Source: CAD feature listing. Evaluate the final solid. Frame: model axes, mm. Face numbers are marked on the shaded views. Round coordinates to 2 decimals unless told otherwise and drop trailing zeros. Write each loop counter-clockwise with the first axis right and the second up, starting at its lowest first coordinate (ties: lowest second). Pieces come first, ordered by that corner, then holes. Notation, with made-up numbers: M 78.5,67.25 L 91.5,67.25 A12 cw 91.5,75.25 Z; hole C 49.25,20.5 d3. An arc over 180 degrees is marked long. Answer in a Markdown table with one row per item. Add a question column.
Item 1: Cut plane B-B on y = 7.5. Return loops of the section in (x, z), and give its area (3 significant figures).
Item 2: Cut plane A-A on x = 29. Return loops of the section in (y, z).
Item 3: Mould query, pull axis Y, two halves, no side actions, for the marked faces 1, 2 and 3. Classes: released by +Y, released by -Y, zero draft, split by the parting line, or undercut.
Item 4: Material intervals for probe 1 along X at (y, z) = (-14, 21.25); probe 2 along Z at (x, y) = (-7, -21.5); probe 3 along Y at (x, z) = (20.5, 21), sorted ascending.
from build123d import *

# Parameters (mm, degrees)
SUPPORT_PLANE_EXACTLY_20MM_ABOVE_TABLE_DEPTH   = 20
LOW_LOCATING_LIP_0P4MM_CLEARANCE_EACH_SI_START = 20
LOW_LOCATING_LIP_0P4MM_CLEARANCE_EACH_SI_DEPTH = 2


with BuildPart() as part:
    # 草图1 → Support_plane_exactly_20mm_above_table (new body)
    with BuildSketch(Plane.XY):
        Polygon((-38.4, -30.7095), (38.4, -30.7095), (41.4, -27.7095), (41.4, 27.7095), (38.4, 30.7095), (-38.4, 30.7095), (-41.4, 27.7095), (-41.4, -27.7095), align=None)
    extrude(amount=SUPPORT_PLANE_EXACTLY_20MM_ABOVE_TABLE_DEPTH)

    # 草图2 → Low_locating_lip_0p4mm_clearance_each_side (add)
    with BuildSketch(Plane.XY.offset(LOW_LOCATING_LIP_0P4MM_CLEARANCE_EACH_SI_START)):
        Polygon((-38.4, -30.7095), (38.4, -30.7095), (41.4, -27.7095), (41.4, 27.7095), (38.4, 30.7095), (-38.4, 30.7095), (-41.4, 27.7095), (-41.4, -27.7095), align=None)
        Polygon((-35.4, -27.7095), (35.4, -27.7095), (38.4, -24.7095), (38.4, 24.7095), (35.4, 27.7095), (-35.4, 27.7095), (-38.4, 24.7095), (-38.4, -24.7095), align=None, mode=Mode.SUBTRACT)
    extrude(amount=LOW_LOCATING_LIP_0P4MM_CLEARANCE_EACH_SI_DEPTH)


solid = part.part
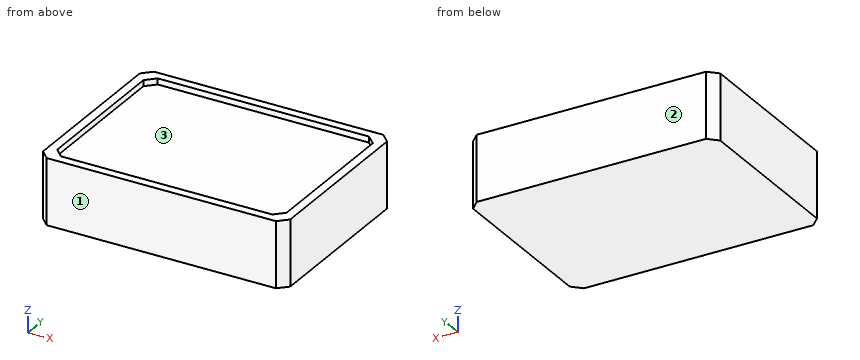
Results below:
| question | item | result |
|---|---|---|
| 1 | outline | M -41.4,0 L 41.4,0 L 41.4,22 L 38.4,22 L 38.4,20 L -38.4,20 L -38.4,22 L -41.4,22 Z |
| 1 | area | 1,670 mm2 |
| 2 | outline | M -30.71,0 L 30.71,0 L 30.71,22 L 27.71,22 L 27.71,20 L -27.71,20 L -27.71,22 L -30.71,22 Z |
| 3 | face 1 | released by -Y |
| 3 | face 2 | released by +Y |
| 3 | face 3 | undercut |
| 4 | probe 1 | -41.4 to -38.4, 38.4 to 41.4 |
| 4 | probe 2 | 0 to 20 |
| 4 | probe 3 | -30.71 to -27.71, 27.71 to 30.71 |
